Part model, mm, in its own coordinate system. A direction names the side the tool comes from. Round coordinates to 2 decimals unless told otherwise and drop trailing zeros. Order: outer loops, then holes, each group sorted by start corner. A loop starts at its lowest first (then second) coordinate and runs counter-clockwise, first axis right, second up. Notation, with made-up numbers: (-19, 84.25) -> (23, 84.25) arc R32 cw to (23, 122.25) -> close; hole circle Ø5 at (64, 74.25). An arc over 180 degrees is marked (long way). Use CSV: the item, a comma, the result in double quotes.
Autodesk Inventor part; units mm, degrees
ref_plane "YZ Plane" through (0, 0, 0) normal (1, 0, 0) x (0, 1, 0)
ref_plane "XZ Plane" through (0, 0, 0) normal (0, 1, 0) x (-1, 0, 0)
ref_plane "XY Plane" through (0, 0, 0) normal (0, 0, 1) x (1, 0, 0)
sketch "Sketch1" plane through (0, 0, 0) normal (0, 0, 1) x (1, 0, 0)
  line L0 (-18.83, -25) -> (18.83, -25)
  line L1 (25, -18.83) -> (25, 18.83)
  line L2 (18.83, 25) -> (-18.83, 25)
  line L3 (-25, 18.83) -> (-25, -18.83)
  line L4 (-25, -25) -> (25, 25) construction
  line L5 (25, -25) -> (-25, 25) construction
  circle A0 centre (0, 0) radius 2.51
  circle A1 centre (0, 10) radius 2.51
  circle A2 centre (-10, 0) radius 2.51
  circle A3 centre (0, -10) radius 2.51
  circle A4 centre (10, 0) radius 2.51
  arc A5 (-18.83, 25) -> (-25, 18.83) centre (-18.83, 18.83) ccw
  arc A6 (25, 18.83) -> (18.83, 25) centre (18.83, 18.83) ccw
  arc A7 (18.83, -25) -> (25, -18.83) centre (18.83, -18.83) ccw
  arc A8 (-25, -18.83) -> (-18.83, -25) centre (-18.83, -18.83) ccw
  dimension "d0" = 50
  dimension "d1" = 50
  dimension "d2" = 5.02
  dimension "d3" = 5.02
  dimension "d6" = 360
  dimension "d8" = 10
  dimension "d9" = 6.17
extrude "Extrusion1" add sketch "Sketch1" along normal mid plane 6.35
sketch "Sketch2" plane through (0, 0, 3.175) normal (0, 0, 1) x (1, 0, 0)
  circle A0 centre (15, 15) radius 5
  circle A1 centre (15, 15) radius 2.5
  point P0 (0, 0)
  dimension "d18" = 10
  dimension "d19" = 5
  dimension "d20" = 15
  dimension "d21" = 15
extrude "Extrusion3" cut sketch "Sketch2" against normal blind 1.625 contours A0 | A1
extrude "Extrusion4" cut sketch "Sketch2" against normal through all contours A1
mirror "Mirror1" about plane through (0, 0, 0) normal (1, 0, 0) of "Extrusion3", "Extrusion4"
mirror "Mirror2" about plane through (0, 0, 0) normal (0, 1, 0) of "Extrusion3", "Extrusion4", "Mirror1"
properties part number "vwheel_plate" material "Aluminum 6061"
(1) Cut at C-C, the plane z = -0.5. State how many separate pieces and enclosed holes the cut face has, then the cut area to 3 significant figures.
Reply:
separate pieces,"1"
enclosed holes,"9"
area,"2,290 mm2"
(2) Probe probe 1 along Y at (x, z) = (-15, -0.15); probe 2 along Y at (x, z) = (15, 2.6). List the from-to ranges inside material, lowest first. Write a range as [from, to].
Reply:
probe 1,"[-25, -17.5], [-12.5, 12.5], [17.5, 25]"
probe 2,"[-25, -20], [-10, 10], [20, 25]"
(3) Drop flat-ended pins along their axis: P1, Ø4.5, axis at x = 15, y = -15, coming from the +Z side; P2, Ø6, axis at x = -15, y = 15, coming from the +Z side. Give the stop position or say it passes through.
Reply:
P1,"through"
P2,"z = 1.55"
(4) Pull direction X, two halves, no side cores. Call faces 3 (the face through (-0.54, -7.55, -0.04)), 4 (the face through (-23.241, 23.145, -0.044)), 5 (the face through (0, 6, 3.175)): released by +X, released by -X, zero draft, split by the parting line, or undercut.
Reply:
face 3,"undercut"
face 4,"released by -X"
face 5,"zero draft"
(5) Cut at A-A, the plane x = 0. Give the cut face in (y, z) (3 decimals).
Reply:
outline,"(-25, -3.175) -> (-12.51, -3.175) -> (-12.51, 3.175) -> (-25, 3.175) -> close; (-7.49, -3.175) -> (-2.51, -3.175) -> (-2.51, 3.175) -> (-7.49, 3.175) -> close; (2.51, -3.175) -> (7.49, -3.175) -> (7.49, 3.175) -> (2.51, 3.175) -> close; (12.51, -3.175) -> (25, -3.175) -> (25, 3.175) -> (12.51, 3.175) -> close"
(6) Cut at D-D, the plane y = 15. Give the cut face in (x, z) (3 decimals).
Reply:
outline,"(-25, -3.175) -> (-17.5, -3.175) -> (-17.5, 1.55) -> (-20, 1.55) -> (-20, 3.175) -> (-25, 3.175) -> close; (-12.5, -3.175) -> (12.5, -3.175) -> (12.5, 1.55) -> (10, 1.55) -> (10, 3.175) -> (-10, 3.175) -> (-10, 1.55) -> (-12.5, 1.55) -> close; (17.5, -3.175) -> (25, -3.175) -> (25, 3.175) -> (20, 3.175) -> (20, 1.55) -> (17.5, 1.55) -> close"
(7) Which spindle directions (+Z, -Z, +X, -X, +Y, -Y) get a long thin tool onto all of the face, cutting with end or side? Do faces 1 (the face through (17.307, 10.564, 2.374)), 2 (the face through (12.5, -14.9, -0.8)). Say none if no direction does.
Reply:
face 1,"+Z"
face 2,"+Z, -Z"
